Geometry check sheet. Reference: the model listing, model coordinates, mm. Give positions to 0.01 mm unless a question says otherwise; leave off trailing zeros. Loops run counter-clockwise (first coordinate to the right, second up) from the corner with the lowest first, then second, coordinate; pieces in that order, holes last. Notation, with made-up numbers: (21.5, -23.5) - (45.5, -23.5) arc R33 ccw to (45.5, 15.5) - close; hole circle Ø9 at (41, 75.25). An arc over 180 degrees is marked (long way). Use a Markdown table: item, result. Add a question column.
1. Depth check by flat-ended pin: P1, Ø1, axis at y = 3.5, z = 0, coming from the -X side; P2, Ø1.5, axis at x = 23.5, z = -16.5, coming from the -Y side; P3, Ø1, axis at y = 7.5, z = -5, coming from the +X side; P4, Ø1.5, axis at y = 3.5, z = -29.5, coming from the +X side. Enter the tip coordinate at first touch or a pass-through.
2. Cross-section at B-B on z = 17. Enter the section's corners in (x, y), and give its area (3 significant figures).
3. Material ranges on L1, parallel to Y at x = -46.5, z = -9; L2, parallel to Z at x = -26, y = 8.25; L3, parallel to X at y = 2.75, z = -46, recorded low to high.
4. Draft check along X on faces 1 (the flat face through (0, 4, 51.962)), 2 (the flat face through (0.52, 3.94, -44.88)), 3 (the cylindrical face through (25.12, 4.06, -48.28)), 4 (the flat face through (45.19, 3.94, -25.65)). Enter one of: pulls with the +X half, pulls with the -X half, needs draft (parallel to the pull), parting line crosses it, or undercut.
5. Cross-section at A-A on x = -11. Enter the section's corners in (y, z), and give its area (3 significant figures).
from build123d import *

# Parameters (mm, degrees)
BOSS_EXTRUDE1_DEPTH = 8
CHAMFER1_SIZE       = 10
CHAMFER1_SIZE_2     = 11.917535926
SKETCH4_R           = 2.3
CUT_EXTRUDE1_DEPTH  = 101.029376687
SKETCH7_R           = 2.3
CUT_EXTRUDE2_DEPTH  = 97.338690096
SKETCH6_R           = 2.3
CUT_EXTRUDE3_DEPTH  = 101.029376687
BOSS_EXTRUDE2_START = 5
SKETCH8_R           = 3.3
SKETCH8_R_2         = 2.3
BOSS_EXTRUDE2_DEPTH = 5
BOSS_EXTRUDE3_START = 5
SKETCH9_R           = 3.3
SKETCH9_R_2         = 2.3
BOSS_EXTRUDE3_DEPTH = 5
BOSS_EXTRUDE4_START = 5
SKETCH10_R          = 3.3
SKETCH10_R_2        = 2.3
BOSS_EXTRUDE4_DEPTH = 5
CHAMFER2_SIZE       = 0.5


with BuildPart() as part:
    # Sketch1 → Boss-Extrude1 (new body)
    with BuildSketch(Plane(origin=(0, 0, 0), x_dir=(1, 0, 0), z_dir=(0, 1, 0))):
        Polygon((-60, 0), (-30, -51.961524227), (30, -51.961524227), (60, 0), (30, 51.961524227), (-30, 51.961524227), align=None)
    extrude(amount=BOSS_EXTRUDE1_DEPTH)

    # Chamfer1
    # the kernel refuses this chamfer: 11.917535926, 10 mm, written as the material it takes off along each edge
    with BuildSketch(Plane(origin=(60.716329832, 8, -51.961524227), x_dir=(0, -0.9993728857116146, -0.0354095369136628), z_dir=(-1, 0, 0)), Plane(origin=(-75.358164916, 8, -26.601121946), x_dir=(-0.030665558503474466, -0.9993728857116146, 0.017704768456831187), z_dir=(0.4999999999999998, 0, 0.8660254037844388)), Plane(origin=(14.641835084, 8, 78.562646173), x_dir=(0.03066555850347504, -0.9993728857116146, 0.017704768456831523), z_dir=(0.4999999999999999, 0, -0.8660254037844388))) as chamfer1_piece_1:
        Polygon((CHAMFER1_SIZE * 0.999372885712, CHAMFER1_SIZE * 0.0354095369137), (-CHAMFER1_SIZE_2 * 0.0354095369135, CHAMFER1_SIZE_2 * 0.999372885707), (0, 0), align=None)
    extrude(amount=121.432659665, mode=Mode.SUBTRACT)

    # Sketch4 → Cut-Extrude1 (cut, through all)
    with BuildSketch(Plane(origin=(17.740047471, 24.412407781, 10.242221183), x_dir=(0.8301060005968417, -0.4979011414928852, -0.2510348204397117), z_dir=(0.5566703992264165, 0.766044443118981, 0.3213938048432679))):
        with Locations(Location((41.75562393, 0.929232239, 0), (0, 0, 164.627134315))):
            Circle(SKETCH4_R)
        with Locations(Location((7.440666851, -41.097835456, 0), (0, 0, 164.627134315))):
            Circle(SKETCH4_R)
    extrude(amount=-CUT_EXTRUDE1_DEPTH, mode=Mode.SUBTRACT)

    # Sketch7 → Cut-Extrude2 (cut, through all)
    with BuildSketch(Plane(origin=(0, 24.412407781, -20.484442365), x_dir=(1, 0, 0), z_dir=(0, 0.7660444431189811, -0.6427876096865357))):
        with Locations(Location((-27.128355545, 31.756069148, 0), (0, 0, 270))):
            Circle(SKETCH7_R)
        with Locations(Location((27.128355545, 31.756069148, 0), (0, 0, 270))):
            Circle(SKETCH7_R)
    extrude(amount=-CUT_EXTRUDE2_DEPTH, mode=Mode.SUBTRACT)

    # Sketch6 → Cut-Extrude3 (cut, through all)
    with BuildSketch(Plane(origin=(-17.740047471, 24.412407781, 10.242221183), x_dir=(0.8307334510088673, 0.5133226132381532, 0.21536440772154375), z_dir=(-0.5566703992264166, 0.766044443118981, 0.3213938048432678))):
        with Locations(Location((-41.687976983, 2.551112975, 0), (0, 0, 193.145847187))):
            Circle(SKETCH6_R)
        with Locations(Location((-9.032068506, -40.777657373, 0), (0, 0, 193.145847187))):
            Circle(SKETCH6_R)
    extrude(amount=-CUT_EXTRUDE3_DEPTH, mode=Mode.SUBTRACT)

    # Sketch8 → Boss-Extrude2 (add)
    # profile 1 of 2: a face of its own
    with BuildSketch(Plane(origin=(17.740047471, 24.412407781, 10.242221183), x_dir=(0.8307334510088674, -0.5133226132381531, -0.21536440772154372), z_dir=(0.5566703992264164, 0.766044443118981, 0.32139380484326796)).offset(BOSS_EXTRUDE2_START)):
        with Locations(Location((9.032068506, -40.777657373, 0), (0, 0, 166.854152813))):
            Circle(SKETCH8_R)
        with Locations(Location((9.032068506, -40.777657373, 0), (0, 0, 166.854152813))):
            Circle(SKETCH8_R_2, mode=Mode.SUBTRACT)
    # profile 2 of 2: a face of its own
    with BuildSketch(Plane(origin=(17.740047471, 24.412407781, 10.242221183), x_dir=(0.8307334510088674, -0.5133226132381531, -0.21536440772154372), z_dir=(0.5566703992264164, 0.766044443118981, 0.32139380484326796)).offset(BOSS_EXTRUDE2_START)):
        with Locations(Location((41.687976983, 2.551112975, 0), (0, 0, 166.854152813))):
            Circle(SKETCH8_R)
        with Locations(Location((41.687976983, 2.551112975, 0), (0, 0, 166.854152813))):
            Circle(SKETCH8_R_2, mode=Mode.SUBTRACT)
    extrude(amount=-BOSS_EXTRUDE2_DEPTH)

    # Sketch9 → Boss-Extrude3 (add)
    # profile 1 of 2: a face of its own
    with BuildSketch(Plane(origin=(-17.740047471, 24.412407781, 10.242221183), x_dir=(0.8307334510088673, 0.5133226132381532, 0.21536440772154375), z_dir=(-0.5566703992264166, 0.766044443118981, 0.3213938048432678)).offset(BOSS_EXTRUDE3_START)):
        with Locations(Location((-41.687976983, 2.551112975, 0), (0, 0, 193.145847187))):
            Circle(SKETCH9_R)
        with Locations(Location((-41.687976983, 2.551112975, 0), (0, 0, 193.145847187))):
            Circle(SKETCH9_R_2, mode=Mode.SUBTRACT)
    # profile 2 of 2: a face of its own
    with BuildSketch(Plane(origin=(-17.740047471, 24.412407781, 10.242221183), x_dir=(0.8307334510088673, 0.5133226132381532, 0.21536440772154375), z_dir=(-0.5566703992264166, 0.766044443118981, 0.3213938048432678)).offset(BOSS_EXTRUDE3_START)):
        with Locations(Location((-9.032068506, -40.777657373, 0), (0, 0, 193.145847187))):
            Circle(SKETCH9_R)
        with Locations(Location((-9.032068506, -40.777657373, 0), (0, 0, 193.145847187))):
            Circle(SKETCH9_R_2, mode=Mode.SUBTRACT)
    extrude(amount=-BOSS_EXTRUDE3_DEPTH)

    # Sketch10 → Boss-Extrude4 (add)
    # profile 1 of 2: a face of its own
    with BuildSketch(Plane(origin=(0, 24.412407781, -20.484442365), x_dir=(1, 0, 0), z_dir=(0, 0.7660444431189811, -0.6427876096865357)).offset(BOSS_EXTRUDE4_START)):
        with Locations(Location((-27.128355545, 31.756069148, 0), (0, 0, 270))):
            Circle(SKETCH10_R)
        with Locations(Location((-27.128355545, 31.756069148, 0), (0, 0, 270))):
            Circle(SKETCH10_R_2, mode=Mode.SUBTRACT)
    # profile 2 of 2: a face of its own
    with BuildSketch(Plane(origin=(0, 24.412407781, -20.484442365), x_dir=(1, 0, 0), z_dir=(0, 0.7660444431189811, -0.6427876096865357)).offset(BOSS_EXTRUDE4_START)):
        with Locations(Location((27.128355545, 31.756069148, 0), (0, 0, 270))):
            Circle(SKETCH10_R)
        with Locations(Location((27.128355545, 31.756069148, 0), (0, 0, 270))):
            Circle(SKETCH10_R_2, mode=Mode.SUBTRACT)
    extrude(amount=-BOSS_EXTRUDE4_DEPTH)

    # Chamfer2
    chamfer2_edges = [part.edges().sort_by_distance(p)[0] for p in [
        (27.128355545, 5.709023104, -50.552887382),
        (30.696220434, 5.890287901, 47.506315425),
        (57.824575979, 5.890287901, 0.518625295),
        (-52.485416923, 9.77015653, 0.518625295),
        (-25.357061378, 9.77015653, 47.506315425),
        (-27.128355545, 5.709023104, -50.552887382),
    ]]
    chamfer(chamfer2_edges, length=CHAMFER2_SIZE)


solid = part.part
Values found:
| question | item | result |
|---|---|---|
| 1 | P1 | stops at x = -56.44 |
| 1 | P2 | stops at y = 0 |
| 1 | P3 | stops at x = 50.56 |
| 1 | P4 | stops at x = 43.4 |
| 2 | outline | (-47.43, 0) - (47.43, 0) - (36.42, 8) - (-36.42, 8) - close |
| 2 | area | 671 mm2 |
| 3 | L1 | y = 0 to 8 |
| 3 | L2 | z = -45.76 to -44.33, 44.36 to 45.83, 48.61 to 49.59 |
| 3 | L3 | x = -33.44 to -28.66, -25.6 to 25.6, 28.66 to 33.44 |
| 4 | face 1 | needs draft |
| 4 | face 2 | undercut |
| 4 | face 3 | undercut |
| 4 | face 4 | pulls with the +X half |
| 5 | outline | (0, -49.58) - (8, -40.04) - (8, 51.96) - (0, 51.96) - close |
| 5 | area | 774 mm2 |
